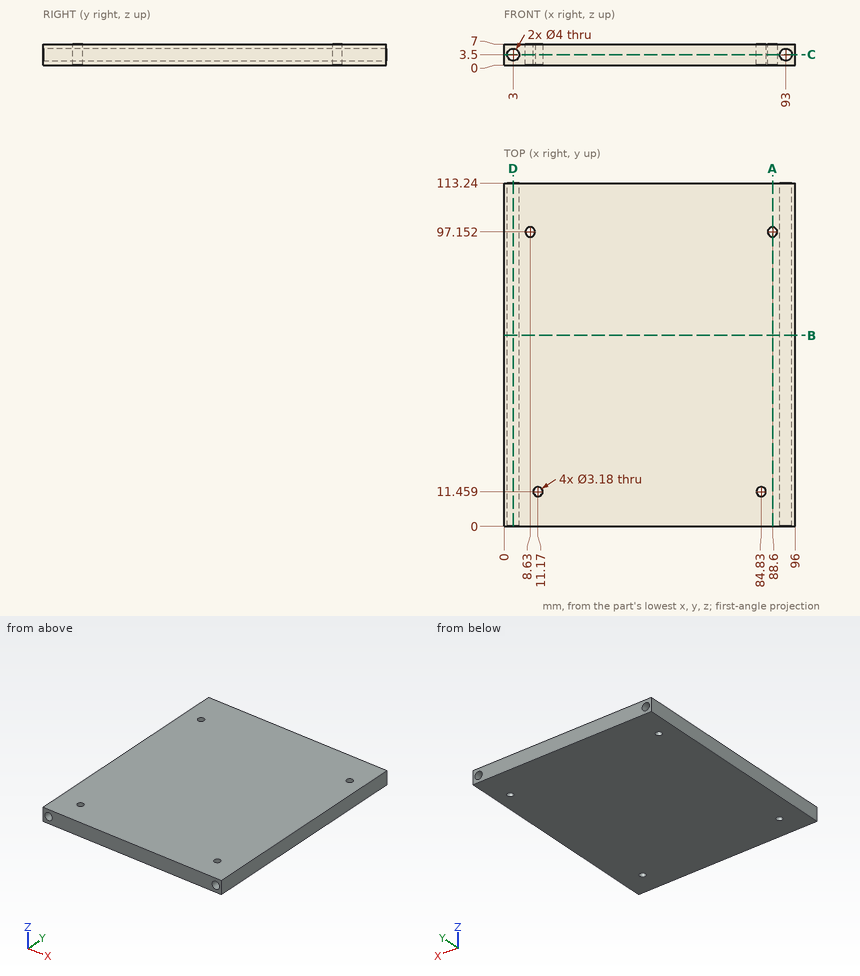
Verification items for this drawing (mm, ordinates from the low corner). Give positions to 0.01 mm unless a question says otherwise; leave off trailing zeros. Write each loop counter-clockwise with the first axis right and the second up, starting at its lowest first coordinate (ties: lowest second). Pieces come first, ordered by that corner, then holes. Notation, with made-up numbers: (13, 74) - (47, 74) arc R28 ccw to (47, 112) - close; hole circle Ø11 at (28, -6). An arc over 180 degrees is marked (long way). Answer as a JSON object with one key per item and string values. Group by question number.
1) Sectioned sample at A-A (x = 88.6). Record the cut outline in (y, z).
2) Sectioned sample at C-C (z = 3.5). Record the cut outline in (x, y), then the cut area to 3 significant figures.
3) Sectioned sample at D-D (x = 3). Record the cut outline in (y, z).
4) Depth check by flat-ended pin: P1, Ø1.9, axis at x = 11.17, y = 11.46, coming from the -Z side. Enter the tip coordinate at first touch or a pass-through.
5) Thickness scan on probe 1 along X at (y, z) = (85, 3.75) (1 decimal); probe 2 along Z at (x, y) = (3, 42.5); probe 3 along Y at (x, z) = (11.17, 1.5). Record the ranges inside material, lowest first. Write a range as from..to.
6) Sectioned sample at B-B (y = 63). Record the cut outline in (x, z).
Geometry results:
{
 "1": {"outline": "(0, 0) - (95.56, 0) - (95.56, 7) - (0, 7) - close; (98.74, 0) - (113.24, 0) - (113.24, 7) - (98.74, 7) - close"},
 "2": {"outline": "(0, 0) - (1, 0) - (1, 113.24) - (0, 113.24) - close; (5, 0) - (91, 0) - (91, 113.24) - (5, 113.24) - close; (95, 0) - (96, 0) - (96, 113.24) - (95, 113.24) - close; hole circle Ø3.18 at (8.63, 97.15); hole circle Ø3.18 at (11.17, 11.46); hole circle Ø3.18 at (84.83, 11.46); hole circle Ø3.18 at (88.6, 97.15)", "area": "9,930 mm^2"},
 "3": {"outline": "(0, 0) - (113.24, 0) - (113.24, 1.5) - (0, 1.5) - close; (0, 5.5) - (113.24, 5.5) - (113.24, 7) - (0, 7) - close"},
 "4": {"P1": "passes through"},
 "5": {"probe 1": "x = 0..1, 5..91, 95..96", "probe 2": "z = 0..1.5, 5.5..7", "probe 3": "y = 0..9.87, 13.05..113.24"},
 "6": {"outline": "(0, 0) - (96, 0) - (96, 7) - (0, 7) - close; hole circle Ø4 at (3, 3.5); hole circle Ø4 at (93, 3.5)"}
}
